Geometry: final body of the model. Coordinates: model frame, mm. Face numbers are marked on the shaded views. A direction names the side the tool comes from. Round coordinates to 2 decimals unless told otherwise and drop trailing zeros. Use one line per item in the form item = value. Start each with the question number.
Item 1: Pull-direction query (X, two-part tool) for the marked faces 6, 7, 8 and 9; classes: pulls with the +X half, pulls with the -X half, needs draft (parallel to the pull), parting line crosses it, or undercut.
Item 2: Ray query, probe 1 along Z at (x, y) = (6, 3.85); probe 2 along Z at (x, y) = (56, 1.7); probe 3 along X at (y, z) = (0.95, -13.5). Return the intervals inside material, ascending.
Item 3: Reachability of the marked faces 1, 2, 3, 4 and 5 from +Z, -Z, +X, -X, +Y, -Y: full face, straight path, thin tool, end or side. Return the list, or none.
Item 4: Section query A-A (y = 2.4). State how many separate pieces and enclosed holes the cut face has, and give its area (3 significant figures).
Item 5: Pin query (flat end, axial travel): pin 1 Ø2 at (x, z) = (31.5, -42) entering from -Y; pin 2 Ø1.3 at (x, y) = (30.5, 2.5) entering from -Z; pin 3 Ø1.3 at (x, y) = (31, 2.5) entering from +Z; pin 4 Ø3.5 at (x, z) = (24.95, -43.13) entering from +Y. Return the tip coordinate at first contact, or that it passes through.
from build123d import *

# Parameters (mm, degrees)
BOSS_EXTRUDE1_DEPTH = 4
CUT_EXTRUDE1_REACH  = 6
SKETCH3_R           = 4
SKETCH3_R_2         = 1.7
SKETCH4_R           = 3
CUT_EXTRUDE2_DEPTH  = 4
CIRPATTERN1_COUNT   = 8


with BuildPart() as part:
    # Sketch2 → Boss-Extrude1 (new body)
    with BuildSketch(Plane(origin=(0, 0, 0), x_dir=(1, 0, 0), z_dir=(0, 1, 0))):
        Polygon((52.538734218, 31.842538875), (52.966809318, 31.892862657), (55.345625477, 31.426126758), (58.18102676, 29.953783051), (58.18102676, 28.584463126), (55.345625477, 27.112119419), (52.966809318, 26.64538352), (52.538734218, 26.695707302), (52.101156541, 24.214732135), (52.520808121, 24.115596779), (54.59638672, 22.863553353), (56.757494627, 20.510006991), (56.289031474, 19.223191192), (53.12080355, 18.809586915), (50.72600436, 19.184530393), (50.340910107, 19.378265245), (49.081307935, 17.196423401), (49.441564779, 16.959924277), (50.963799881, 15.07332886), (52.189708735, 12.122809954), (51.309369324, 11.073573865), (48.190601939, 11.768601179), (46.068586453, 12.939866968), (45.772908404, 13.25368769), (43.842900517, 11.634261062), (44.100782542, 11.288690853), (44.885873492, 8.995402472), (45.028637129, 5.803632771), (43.842684706, 5.118756998), (41.149615437, 6.838398802), (39.556106805, 8.664951285), (39.385697153, 9.061061087), (37.018327401, 8.199295971), (37.142300931, 7.786339893), (37.095648999, 5.362815632), (36.138204566, 2.314673579), (34.789402002, 2.076878058), (32.847083699, 4.613576876), (31.97451961, 6.875115771), (31.949681435, 7.305566323), (29.430477092, 7.305566323), (29.405639683, 6.875115771), (28.533075594, 4.613576876), (26.590757291, 2.076878058), (25.241954726, 2.314673579), (24.284510294, 5.362815632), (24.237858361, 7.786339893), (24.361831127, 8.199295971), (21.994461374, 9.061061087), (21.824052488, 8.664951285), (20.230543856, 6.838398802), (17.537474587, 5.118756998), (16.351521398, 5.803632771), (16.494285035, 8.995402472), (17.279376751, 11.288690853), (17.537258011, 11.634261062), (15.607250889, 13.25368769), (15.311572074, 12.939866968), (13.189557354, 11.768601179), (10.070789203, 11.073573865), (9.190449792, 12.122809954), (10.416359412, 15.07332886), (11.938594514, 16.959924277), (12.298851357, 17.196423401), (11.039249186, 19.378265245), (10.654154168, 19.184530393), (8.259354977, 18.809586915), (5.091127819, 19.223191192), (4.622664666, 20.510006991), (6.783771808, 22.863553353), (8.859351172, 24.115596779), (9.279002752, 24.214732135), (8.84142431, 26.695707302), (8.413349975, 26.64538352), (6.034533051, 27.112119419), (3.199132533, 28.584463126), (3.199132533, 29.953783051), (6.034533051, 31.426126758), (8.413349975, 31.892862657), (8.84142431, 31.842538875), (9.279002752, 34.323514042), (8.859351172, 34.422649398), (6.783771808, 35.674692824), (4.622664666, 38.028239186), (5.091127819, 39.315054985), (8.259354977, 39.728659262), (10.654154168, 39.353715784), (11.039249186, 39.159980932), (12.298851357, 41.341822776), (11.938594514, 41.5783219), (10.416359412, 43.464917317), (9.190449792, 46.415436223), (10.070789203, 47.464672312), (13.189557354, 46.769644998), (15.311572074, 45.598379209), (15.607250889, 45.284558487), (17.537258011, 46.903985115), (17.279376751, 47.249555324), (16.494285035, 49.542843705), (16.351521398, 52.734613406), (17.537474587, 53.41948918), (20.230543856, 51.699847375), (21.824052488, 49.873294892), (21.994461374, 49.47718509), (24.361831127, 50.338950206), (24.237858361, 50.751906284), (24.284510294, 53.175430545), (25.241954726, 56.223572598), (26.590757291, 56.46136812), (28.533075594, 53.924669301), (29.405639683, 51.663130406), (29.430477092, 51.232679854), (31.949681435, 51.232679854), (31.97451961, 51.663130406), (32.847083699, 53.924669301), (34.789402002, 56.46136812), (36.138204566, 56.223572598), (37.095648999, 53.175430545), (37.142300931, 50.751906284), (37.018327401, 50.338950206), (39.385697153, 49.47718509), (39.556106805, 49.873294892), (41.149615437, 51.699847375), (43.842684706, 53.41948918), (45.028637129, 52.734613406), (44.885873492, 49.542843705), (44.100782542, 47.249555324), (43.842900517, 46.903985115), (45.772908404, 45.284558487), (46.068586453, 45.598379209), (48.190601939, 46.769644998), (51.309369324, 47.464672312), (52.189708735, 46.415436223), (50.963799881, 43.464917317), (49.441564779, 41.5783219), (49.081307935, 41.341822776), (50.340910107, 39.159980932), (50.72600436, 39.353715784), (53.12080355, 39.728659262), (56.289031474, 39.315054985), (56.757494627, 38.028239186), (54.59638672, 35.674692824), (52.520808121, 34.422649398), (52.101156541, 34.323514042), align=None)
    extrude(amount=BOSS_EXTRUDE1_DEPTH)

    # Sketch3 → Cut-Extrude1 (cut, up to next)
    with BuildSketch(Plane(origin=(0, 0, 0), x_dir=(1, 0, 0), z_dir=(0, 1, 0)), mode=Mode.PRIVATE) as cut_extrude1_sk1:
        with Locations((30.690079264, 29.269123089)):
            Circle(SKETCH3_R)
    cut_extrude1_tool1 = extrude(cut_extrude1_sk1.sketch, amount=CUT_EXTRUDE1_REACH, mode=Mode.PRIVATE) & part.part
    add(cut_extrude1_tool1.solids().sort_by_distance((30.690079, 0, -29.269123))[0], mode=Mode.SUBTRACT)
    # Sketch3 → Cut-Extrude1 (cut, up to next)
    with BuildSketch(Plane(origin=(0, 0, 0), x_dir=(1, 0, 0), z_dir=(0, 1, 0)), mode=Mode.PRIVATE) as cut_extrude1_sk2:
        with Locations((18.690079264, 29.269123089)):
            Circle(SKETCH3_R_2)
    cut_extrude1_tool2 = extrude(cut_extrude1_sk2.sketch, amount=CUT_EXTRUDE1_REACH, mode=Mode.PRIVATE) & part.part
    add(cut_extrude1_tool2.solids().sort_by_distance((18.690079, 0, -29.269123))[0], mode=Mode.SUBTRACT)
    # Sketch3 → Cut-Extrude1 (cut, up to next)
    with BuildSketch(Plane(origin=(0, 0, 0), x_dir=(1, 0, 0), z_dir=(0, 1, 0)), mode=Mode.PRIVATE) as cut_extrude1_sk3:
        with Locations((42.690079264, 29.269123089)):
            Circle(SKETCH3_R_2)
    cut_extrude1_tool3 = extrude(cut_extrude1_sk3.sketch, amount=CUT_EXTRUDE1_REACH, mode=Mode.PRIVATE) & part.part
    add(cut_extrude1_tool3.solids().sort_by_distance((42.690079, 0, -29.269123))[0], mode=Mode.SUBTRACT)

    # Sketch4 → Cut-Extrude2 (cut)
    with BuildSketch(Plane(origin=(0, 0, 0), x_dir=(1, 0, 0), z_dir=(0, 1, 0))):
        with Locations((16.831886276, 35.009374574)):
            Circle(SKETCH4_R)
    cut_extrude2 = extrude(amount=CUT_EXTRUDE2_DEPTH, mode=Mode.SUBTRACT)

    # CirPattern1: Cut-Extrude2 ×8 about axis
    cirpattern1_axis = Axis((30.690079264, 0, -29.269123089), (0, 1, 0))
    for i in range(1, CIRPATTERN1_COUNT):
        add(cut_extrude2.rotate(cirpattern1_axis, i * 360 / CIRPATTERN1_COUNT), mode=Mode.SUBTRACT)


solid = part.part
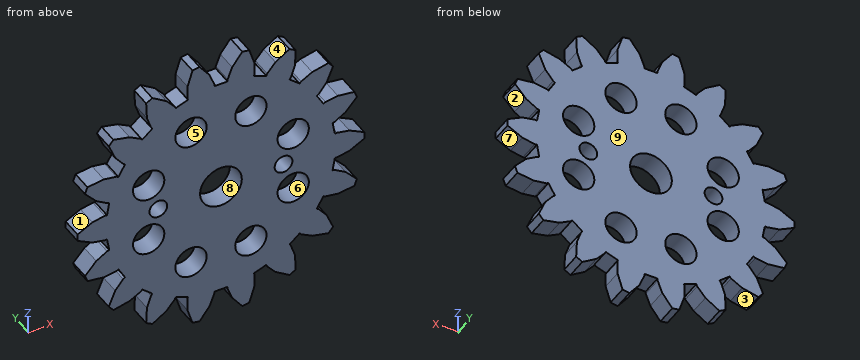
Working result:
q1.face_6 = undercut
q1.face_7 = pulls with the +X half
q1.face_8 = undercut
q1.face_9 = needs draft
q2.probe_1 = -39.43 to -36.53, -31.41 to -27.13, -22.01 to -19.1
q2.probe_2 = -39.35 to -37.2, -31.09 to -27.45, -21.33 to -19.19
q2.probe_3 = 9.76 to 22.64, 27.26 to 34.12, 38.74 to 51.62
q3.face_1 = -X, +Y, -Y
q3.face_2 = +X, +Y, -Y
q3.face_3 = -Z, +Y, -Y
q3.face_4 = +Z, +Y, -Y
q3.face_5 = +Y, -Y
q4.separate_pieces = 1
q4.enclosed_holes = 11
q4.area = 1,610 mm²
q5.pin_1 = 0
q5.pin_2 = -51.23
q5.pin_3 = -7.31
q5.pin_4 = through
